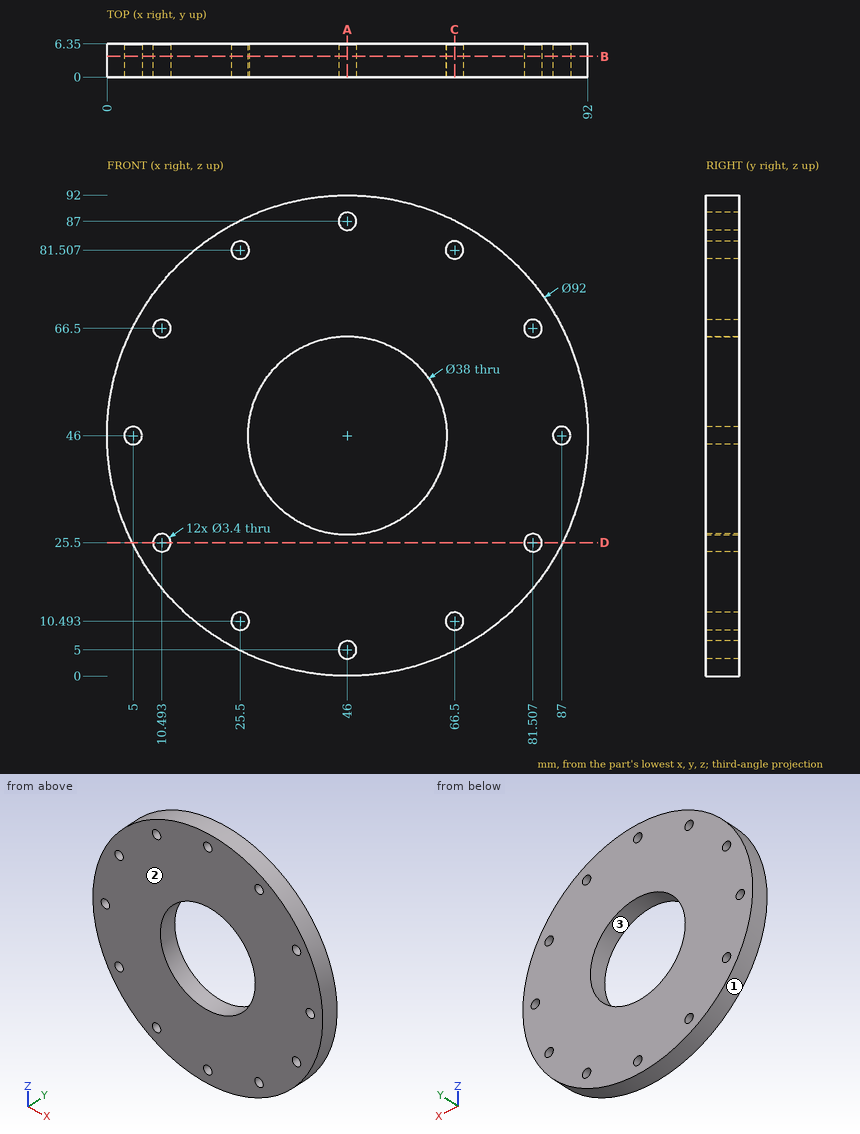
Answer from the drawing. Dimensions are ordinates in mm from the lowest x, y and z of the part. Coordinates: 2 decimals unless noted, no trailing zeros. Write each loop counter-clockwise with the first axis right and the second up, starting at its lowest first coordinate (ties: lowest second). Pieces come first, ordered by that corner, then holes. Notation, with made-up numbers: M 45,-40 L 92,-40 A25 cw 92,-24 Z; hole C 3.5,89.5 d4. An arc over 180 degrees is marked long. Put each result on its own line as item: value. Start each with the question number.
1. A cutting plane is placed at D-D on z = 25.5. Write down the section's boundary in (x, y).
2. A cutting plane is placed at B-B on y = 4. Count the separate pieces of the cut face and the enclosed holes in it, then the cut area to 3 significant figures.
3. A cutting plane is placed at A-A on x = 46. Write down the section's boundary in (y, z).
4. A cutting plane is placed at C-C on x = 66.5. Write down the section's boundary in (y, z), then the cut area to 3 significant figures.
5. For a pull along Z with two mould halves and no side action, classify the marked faces 1, 2 and 3 as pulls with the +Z half, pulls with the -Z half, needs draft (parallel to the pull), parting line crosses it, or undercut.
6. Flat-ended cylindrical pins translate along their axes: P1, Ø3, axis at x = 26.5, y = 2, coming from the +Z side; P2, Ø1, axis at y = 1, z = 43.5, coming from the -X side; P3, Ø1, axis at x = 75, y = 3, coming from the +Z side. Find the tip coordinate at first contact, or state that the pin passes through.
7. Consider line 1 (X direction, y = 2.75, z = 46); line 2 (X direction, y = 1, z = 12); line 3 (X direction, y = 5.75, z = 83). Determine where each line is inside the solid, lowest interval first. Write a range as from..to.
Resolved:
1. outline: M 4.82,0 L 8.79,0 L 8.79,6.35 L 4.82,6.35 Z; M 12.19,0 L 79.81,0 L 79.81,6.35 L 12.19,6.35 Z; M 83.21,0 L 87.18,0 L 87.18,6.35 L 83.21,6.35 Z
2. separate pieces: 1
2. enclosed holes: 13
2. area: 5,400 mm2
3. outline: M 0,0 L 6.35,0 L 6.35,3.3 L 0,3.3 Z; M 0,6.7 L 6.35,6.7 L 6.35,27 L 0,27 Z; M 0,65 L 6.35,65 L 6.35,85.3 L 0,85.3 Z; M 0,88.7 L 6.35,88.7 L 6.35,92 L 0,92 Z
4. outline: M 0,4.82 L 6.35,4.82 L 6.35,8.79 L 0,8.79 Z; M 0,12.19 L 6.35,12.19 L 6.35,79.81 L 0,79.81 Z; M 0,83.21 L 6.35,83.21 L 6.35,87.18 L 0,87.18 Z
4. area: 480 mm2
5. face 1: parting line crosses it
5. face 2: needs draft
5. face 3: undercut
6. P1: stops at z = 88.33
6. P2: stops at x = 0.04
6. P3: stops at z = 82.11
7. line 1: x = 0..3.3, 6.7..27, 65..85.3, 88.7..92
7. line 2: x = 15.02..24.71, 26.29..65.71, 67.29..76.98
7. line 3: x = 18.67..24.69, 26.31..65.69, 67.31..73.33
